Can you work these out from the drawing? Everything is in mm from the part's minimum corner. A direction names the side the tool comes from. Give positions to 0.01 mm unless a question says otherwise; leave off trailing zeros. Order: outer loops, then holes, each group sorted by start corner. A loop starts at its lowest first (then second) coordinate and runs counter-clockwise, first axis right, second up. Notation, with made-up numbers: M 88.25,-26.75 L 132.25,-26.75 A14 ccw 132.25,-0.75 Z; hole C -21.5,-16.75 d11. An arc over 180 degrees is marked long. Use a Markdown table: item, result. Add a question column.
Item 1: Suppose I cut it at A-A on y = 11. Write out the boundary of the cut face in (x, z).
Item 2: I'm going to push flat-ended pins straight in: pin 1 Ø5 at (x, y) = (12.5, 32) entering from +Z; pin 2 Ø8 at (x, y) = (11.5, 31.5) entering from -Z; pin 3 Ø12 at (x, z) = (13.5, 19) entering from -Y; pin 4 Ø9 at (x, z) = (10.5, 27) entering from +Y. Where does each tip first touch, or does it pass through?
Item 3: Suppose I cut it at D-D on x = 7.75. Write out the boundary of the cut face in (y, z) (1 decimal), plus the area to 3 significant figures.
Item 4: Suppose I cut it at B-B on z = 28. Write out the boundary of the cut face in (x, y), plus the area to 3 significant figures.
Item 5: Suppose I cut it at C-C on y = 37.5. Write out the boundary of the cut face in (x, z).
Item 6: If I drill on L1, parallel to X at y = 20, z = 35; L2, parallel to Z at x = 21.5, y = 22; L3, parallel to Z at x = 12.5, y = 13.25, over which ranges is the centre line in solid material (lowest first)? Write a range as from..to.
Item 7: If we mould it in two halves opening along X, with no side actions, what happens to the marked faces 1, 2, 3 and 4? For each: released by +X, released by -X, zero draft, split by the parting line, or undercut.
Item 8: For the marked faces 5 and 6, which set-ups out of +Z, -Z, +X, -X, +Y, -Y let a thin tool reach every point of the face, with its end or its side?
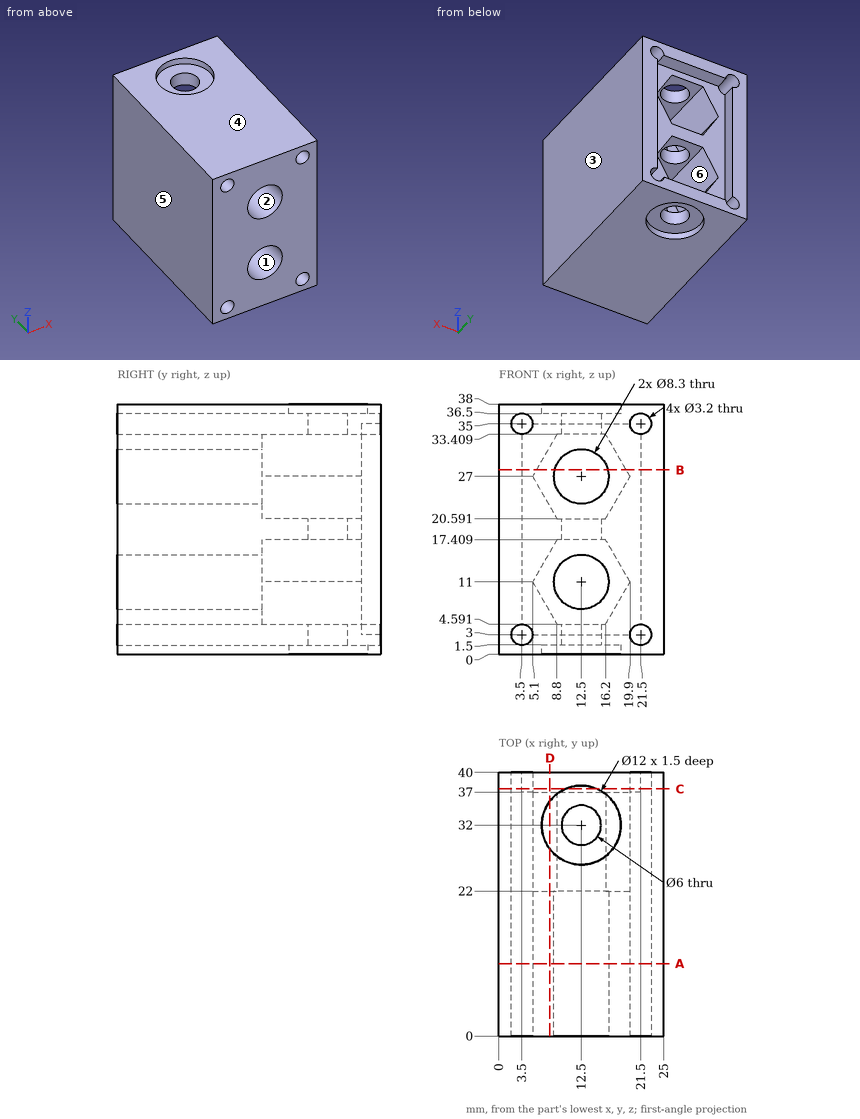
Findings below:
| question | item | result |
|---|---|---|
| 1 | outline | M 0,0 L 25,0 L 25,38 L 0,38 Z; hole C 3.5,3 d3.2; hole C 3.5,35 d3.2; hole C 12.5,11 d8.3; hole C 12.5,27 d8.3; hole C 21.5,3 d3.2; hole C 21.5,35 d3.2 |
| 2 | pin 1 | passes through |
| 2 | pin 2 | stops at z = 1.5 |
| 2 | pin 3 | stops at y = 0 |
| 2 | pin 4 | stops at y = 22 |
| 3 | outline | M 0,0 L 28.3,0 L 28.3,1.5 L 35.7,1.5 L 35.7,0 L 40,0 L 40,3 L 37,3 L 37,6.4 L 22,6.4 L 22,15.6 L 37,15.6 L 37,22.4 L 22,22.4 L 22,31.6 L 37,31.6 L 37,35 L 40,35 L 40,38 L 35.7,38 L 35.7,36.5 L 28.3,36.5 L 28.3,38 L 0,38 Z |
| 3 | area | 1,130 mm^2 |
| 4 | outline | M 0,0 L 8.47,0 L 8.47,22 L 5.68,22 L 5.68,37 L 3.5,37 L 3.5,40 L 0,40 Z; M 16.53,0 L 25,0 L 25,40 L 21.5,40 L 21.5,37 L 19.32,37 L 19.32,22 L 16.53,22 Z |
| 4 | area | 564 mm^2 |
| 5 | outline | M 0,0 L 10.1,0 L 10.1,1.5 L 14.9,1.5 L 14.9,0 L 25,0 L 25,38 L 14.9,38 L 14.9,36.5 L 10.1,36.5 L 10.1,38 L 0,38 Z; hole M 3.5,4.6 A1.6 ccw long 5.1,3 L 19.9,3 A1.6 ccw long 21.5,4.6 L 21.5,33.4 A1.6 ccw long 19.9,35 L 5.1,35 A1.6 ccw long 3.5,33.4 Z |
| 6 | L1 | x = 0..1.9, 5.1..19.9, 23.1..25 |
| 6 | L2 | z = 0..1.4, 4.6..33.4, 36.6..38 |
| 6 | L3 | z = 0..6.85, 15.15..22.85, 31.15..38 |
| 7 | face 1 | undercut |
| 7 | face 2 | undercut |
| 7 | face 3 | released by +X |
| 7 | face 4 | zero draft |
| 8 | face 5 | +Z, -Z, -X, +Y, -Y |
| 8 | face 6 | +Y |
